Read the model definition and answer for the solid it produces. Units are mm, in the model's axes. Face numbers are marked on the shaded views. A direction names the side the tool comes from. Round coordinates to 2 decimals unless told otherwise and drop trailing zeros. Loops run counter-clockwise (first coordinate to the right, second up) from the corner with the lowest first, then second, coordinate; pieces in that order, holes last. Notation, with made-up numbers: (62.5, -31.75) - (116.5, -31.75) arc R12 cw to (116.5, -13.75) - close; hole circle Ø8 at (20.5, -17). An arc over 180 degrees is marked (long way). Use one line per item in the form item = value. Start each with the question number.
```python
from build123d import *

# Parameters (mm, degrees)
BOSS_EXTRUDE1_DEPTH = 5
CUT_EXTRUDE1_DEPTH  = 4
BOSS_EXTRUDE2_DEPTH = 1


with BuildPart() as part:
    # Sketch3 → Boss-Extrude1 (new body)
    with BuildSketch(Plane(origin=(0, 0, 0), x_dir=(0, 0, -1), z_dir=(1, 0, 0))):
        Polygon((1, 2.8), (0, 3.4), (0, 0), (1, 0), align=None)
        Polygon((5, 0), (5, 1), (0, 4), (0, 3.4), (1, 2.8), (4, 1), (4, 0), align=None)
        Polygon((1, 0), (4, 0), (4, 1), (1, 2.8), align=None)
    extrude(amount=BOSS_EXTRUDE1_DEPTH)

    # Sketch3_3 → Cut-Extrude1 (cut)
    with BuildSketch(Plane(origin=(0, 0, 0), x_dir=(0, 0, -1), z_dir=(1, 0, 0))):
        Polygon((1, 0), (4, 0), (4, 1), (1, 2.8), align=None)
    extrude(amount=CUT_EXTRUDE1_DEPTH, mode=Mode.SUBTRACT)

    # Sketch3_4 → Boss-Extrude2 (add)
    with BuildSketch(Plane(origin=(0, 0, 0), x_dir=(0, 0, -1), z_dir=(1, 0, 0))):
        Polygon((1, 0), (4, 0), (4, 1), (1, 2.8), align=None)
    extrude(amount=BOSS_EXTRUDE2_DEPTH)


solid = part.part
```
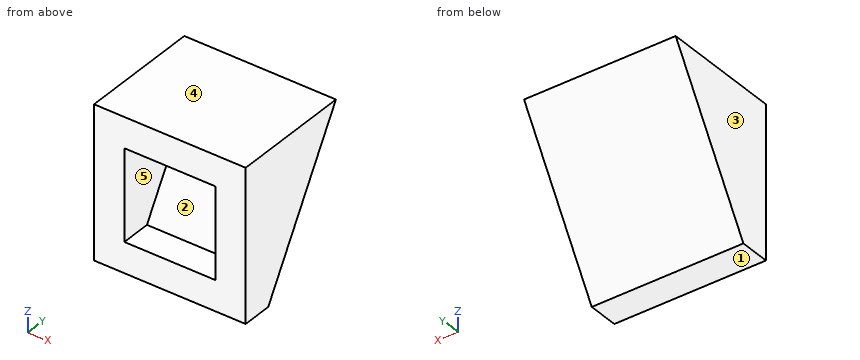
1) For the marked faces 1 and 2, determine the directions among +Z, -Z, +X, -X, +Y, -Y from which every point of the face is accessible in a straight line to the end or side of a thin tool.
2) A cutting plane is placed at D-D on y = 1.1. Write down the section's boundary in (x, z), plus the area to 3 significant figures.
3) A cutting plane is placed at C-C on x = 3. Write down the section's boundary in (y, z), plus the area to 3 significant figures.
4) A flat-ended cylindrical pin translates along its axis: pin 1 (3 mm diameter, centred on x = 3.5, z = -3, fed in from -Y). Find the tip coordinate at first contact, or state that the pin passes through.
5) A cutting plane is placed at B-B on z = -2.2. Write down the section's boundary in (x, y).
6) Determine the mould class of the marked faces 3, 4 and 5 for opening direction X: +X half, -X half, draft (parallel to the pull), parting line (faces both ways), or undercut.
7) A cutting plane is placed at A-A on y = 0.7. Write down the section's boundary in (x, z).
8) Straight lines are drawn through the part: line 1 (X direction, y = 1.4, z = -2.5); line 2 (Z direction, x = 2.8, y = 0.7); line 3 (Y direction, x = 4.1, z = -4.2). For each, find the intervals that lie inside material, in ascending order. Write a range as from..to.
Checks:
q1.face_1 = -Z, +X, -X, +Y, -Y
q1.face_2 = -Y
q2.outline = (0, -4.83) - (5, -4.83) - (5, 0) - (0, 0) - close; hole (1, -3.83) - (4, -3.83) - (4, -1) - (1, -1) - close
q2.area = 15.7 mm²
q3.outline = (0, -5) - (1, -5) - (4, 0) - (0, 0) - (0, -1) - (2.8, -1) - (1, -4) - (0, -4) - close
q3.area = 6.80 mm²
q4.pin_1 = 0
q5.outline = (0, 0) - (1, 0) - (1, 2.08) - (4, 2.08) - (4, 0) - (5, 0) - (5, 2.68) - (0, 2.68) - close
q6.face_3 = -X half
q6.face_4 = draft
q6.face_5 = undercut
q7.outline = (0, -5) - (5, -5) - (5, 0) - (0, 0) - close; hole (1, -4) - (4, -4) - (4, -1) - (1, -1) - close
q8.line_1 = 0..1, 4..5
q8.line_2 = -5..-4, -1..0
q8.line_3 = 0..1.48
